Autodesk Inventor part; units mm, degrees
ref_plane "YZ Plane" through (0, 0, 0) normal (1, 0, 0) x (0, 1, 0)
ref_plane "XZ Plane" through (0, 0, 0) normal (0, 1, 0) x (-1, 0, 0)
ref_plane "XY Plane" through (0, 0, 0) normal (0, 0, 1) x (1, 0, 0)
sketch "Sketch8" plane through (0, 0, 0) normal (0, 0, 1) x (1, 0, 0)
  circle A0 centre (0, 0) radius 15
  dimension "d33" = 30
extrude "Extrusion7" add sketch "Sketch8" against normal blind 8
sketch "Sketch10" plane through (0, 0, -8) normal (0, 0, -1) x (-1, 0, 0)
  line L0 (9, 10.07) -> (-29.1, 10.07)
  arc A0 (10, 9.07) -> (9, 10.07) centre (9, 9.07) ccw
  line L1 (10, 9.07) -> (10, -9.07)
  arc A1 (9, -10.07) -> (10, -9.07) centre (9, -9.07) ccw
  line L2 (-29.1, -10.07) -> (9, -10.07)
  line L3 (-29.1, 10.07) -> (-29.1, -10.07)
  line L4 (10.4, -9.07) -> (10.4, 9.07)
  arc A2 (10.4, 9.07) -> (9, 10.47) centre (9, 9.07) ccw
  line L5 (9, 10.47) -> (-29.5, 10.47)
  line L6 (-29.5, 10.47) -> (-29.5, -10.47)
  line L7 (-29.5, -10.47) -> (9, -10.47)
  arc A3 (9, -10.47) -> (10.4, -9.07) centre (9, -9.07) ccw
  dimension "d59" = 0.4
extrude "Extrusion8" cut sketch "Sketch10" against normal blind 2 contours A0 L1 A1 L2 L3 L0 | A3 L7 L6 L5 A2 L4
sketch "Sketch11" plane through (0, 0, -6) normal (0, 0, -1) x (-1, 0, 0)
  circle A0 centre (0, 0) radius 6.4
  circle A1 centre (0, 0) radius 6.5
  point P0 (0, 0)
  dimension "d58" = 13
extrude "Extrusion9" cut sketch "Sketch11" against normal through all contours A0 | A1
sketch "Sketch13" plane through (0, 0, 0) normal (0, 0, 1) x (1, 0, 0)
  circle A0 centre (0, 0) radius 9.96
  circle A1 centre (0, 0) radius 10.16
  point P0 (0, 0)
  dimension "d44" = 0.2
extrude "Extrusion11" cut sketch "Sketch13" against normal blind 3 contours A0 | A1
sketch "Sketch14" plane through (0, 0, 0) normal (0, 0, 1) x (1, 0, 0)
  circle A0 centre (6.9, 8) radius 0.7835
  circle A1 centre (6.9, -8) radius 0.7835
  circle A2 centre (-8, 8.07) radius 1
  circle A3 centre (-8, -8.07) radius 1
  point P0 (0, 0)
hole "Hole2" at (6.9, 8, 0) at (-8, 8.07, 0) at (-8, -8.07, 0) at (6.9, -8, 0) direction (0, 0, -1) diameter 2.1 end through all
sketch "Sketch15" plane through (0, 0, 0) normal (0, 0, 1) x (1, 0, 0)
  arc A0 (7.3255, 7.0401) -> (5.888, 8.2799) centre (6.9, 8) ccw
  arc A1 (5.888, -8.2799) -> (7.3255, -7.0401) centre (6.9, -8) ccw
  circle A2 centre (-8, 8.07) radius 1.05
  circle A3 centre (-8, -8.07) radius 1.05
  circle A4 centre (6.9, 8) radius 1.9
  circle A5 centre (6.9, -8) radius 1.9
  circle A6 centre (-8, -8.07) radius 1.9
  circle A7 centre (-8, 8.07) radius 1.9
  point P0 (0, 0)
  dimension "d54" = 3.8
extrude "Extrusion12" cut sketch "Sketch15" against normal blind 4.5 contours A2 | A3 | A4 | A5 | A6 | A7
fillet "Fillet2" radius 0.5 8 edges at (5.1562, 8.7544, -1.5) (7.9023, 6.3859, -1.5) (-6.1008, 8.1244, -1.5) (-8.071, 6.1713, -1.5) (-8.071, -6.1713, -1.5) (-6.1008, -8.1244, -1.5) (5.1562, -8.7544, -1.5) (7.9023, -6.3859, -1.5)
sketch "Sketch16" plane through (0, 0, -8) normal (0, 0, -1) x (-1, 0, 0)
  circle A0 centre (-6.9, -8) radius 1.05
  circle A1 centre (8, -8.07) radius 1.05
  circle A2 centre (8, 8.07) radius 1.05
  circle A3 centre (-6.9, 8) radius 1.05
  circle A4 centre (0, 0) radius 6.5
  arc A5 (-10.7415, 10.47) -> (-10.7415, -10.47) centre (0, 0) ccw
  line L0 (9, -10.47) -> (-10.7415, -10.47)
  arc A6 (9, -10.47) -> (10.4, -9.07) centre (9, -9.07) ccw
  line L1 (10.4, 9.07) -> (10.4, -9.07)
  arc A7 (10.4, 9.07) -> (9, 10.47) centre (9, 9.07) ccw
  line L2 (-10.7415, 10.47) -> (9, 10.47)
  line L3 (-10.7415, 10.47) -> (9, 10.47)
  arc A8 (10.4, 9.07) -> (9, 10.47) centre (9, 9.07) ccw
  line L4 (10.4, 9.07) -> (10.4, -9.07)
  arc A9 (9, -10.47) -> (10.4, -9.07) centre (9, -9.07) ccw
  line L5 (9, -10.47) -> (-10.7415, -10.47)
  arc A10 (-10.7415, -10.47) -> (-10.7415, 10.47) centre (0, 0) ccw
sketch "Sketch17" plane through (0, 0, -3) normal (0, 0, 1) x (1, 0, 0)
  circle A0 centre (6.9, 8) radius 1.05
  circle A1 centre (6.9, 8) radius 1.9
  circle A2 centre (6.9, -8) radius 1.05
  circle A3 centre (6.9, -8) radius 1.9
  circle A4 centre (-8, 8.07) radius 1.05
  circle A5 centre (-8, 8.07) radius 1.9
  circle A6 centre (-8, -8.07) radius 1.05
  circle A7 centre (-8, -8.07) radius 1.9
  point P0 (0, 0)
extrude "Extrusion13" add sketch "Sketch17" against normal blind 1.5
extrude "Extrusion14" cut sketch "Sketch16" against normal blind 3.5
properties part number "frame_motor_support_top" material "Aluminum 6061-AHC"
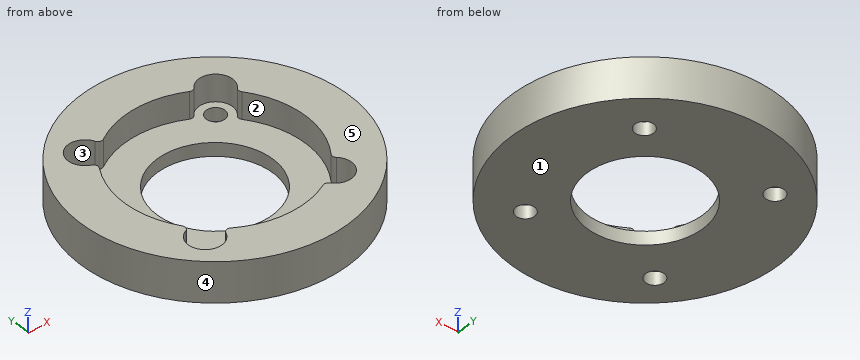
Source: CAD feature listing. Evaluate the final solid. Frame: model axes, mm. Face numbers are marked on the shaded views. A direction names the side the tool comes from. Round coordinates to 2 decimals unless told otherwise and drop trailing zeros. Loops run counter-clockwise (first coordinate to the right, second up) from the corner with the lowest first, then second, coordinate; pieces in that order, holes last. Notation, with made-up numbers: M 86,34 L 119,34 A37 cw 119,71 Z; hole C 66,7 d1. An arc over 180 degrees is marked long. Return JSON: item names as keys, results as strings. Group by question number.
1. Mould query, pull axis X, two halves, no side actions, for the marked faces 3, 4 and 5. Classes: released by +X, released by -X, zero draft, split by the parting line, or undercut.
2. Section query D-D on z = -4.05. Output: boundary loops of the cut face in (x, y).
3. Section query B-B on y = -2.5. Output: boundary loops of the cut face in (x, z), and give its area (3 significant figures).
4. Material intervals for line 1 along Y through (x, z) = (8.5, -0.4); line 2 along Y through (x, z) = (6.9, -3.7); line 3 along Z through (x, y) = (-1.5, 9.5), sorted ascending. Write a range as from..to.
5. Pin query (flat end, axial travel): pin 1 (10 mm diameter, centred on x = -4.5, y = 1.5, fed in from +Z). Return the tip coordinate at first contact, or that it passes through.
6. Section query A-A on x = 0. Output: boundary loops of the cut face in (y, z), and give its area (3 significant figures).
7. Reachability of the marked faces 1 and 2 from +Z, -Z, +X, -X, +Y, -Y: full face, straight path, thin tool, end or side. Return the list, or none.
8. Section query C-C on x = 6.9. Output: boundary loops of the cut face in (y, z).
Checks:
{
 "1": {"face 3": "undercut", "face 4": "split by the parting line", "face 5": "zero draft"},
 "2": {"outline": "C 0,0 d30; hole C -8,-8.07 d2.1; hole C -8,8.07 d2.1; hole C 0,0 d13; hole C 6.9,-8 d2.1; hole C 6.9,8 d2.1"},
 "3": {"outline": "M -14.79,-4.5 L -6,-4.5 L -6,-3 L -9.85,-3 L -9.85,0 L -14.79,0 Z; M 6,-4.5 L 14.79,-4.5 L 14.79,0 L 9.85,0 L 9.85,-3 L 6,-3 Z", "area": "56.0 mm²"},
 "4": {"line 1": "y = -12.36..-9.02, -6.98..-5.57, 5.57..6.98, 9.02..12.36", "line 2": "y = -13.32..-9.05, -6.95..6.95, 9.05..13.32", "line 3": "z = -4.5..-3"},
 "5": {"pin 1": "stops at z = -3"},
 "6": {"outline": "M -15,-4.5 L -6.5,-4.5 L -6.5,-3 L -10.16,-3 L -10.16,0 L -15,0 Z; M 6.5,-4.5 L 15,-4.5 L 15,0 L 10.16,0 L 10.16,-3 L 6.5,-3 Z", "area": "54.5 mm²"},
 "7": {"face 1": "-Z, +X, -X, +Y, -Y", "face 2": "+Z"},
 "8": {"outline": "M -13.32,-4.5 L -9.05,-4.5 L -9.05,-3 L -9.9,-3 L -9.9,0 L -13.32,0 Z; M -6.95,-4.5 L 6.95,-4.5 L 6.95,-3 L -6.95,-3 Z; M 9.05,-4.5 L 13.32,-4.5 L 13.32,0 L 9.9,0 L 9.9,-3 L 9.05,-3 Z"}
}
